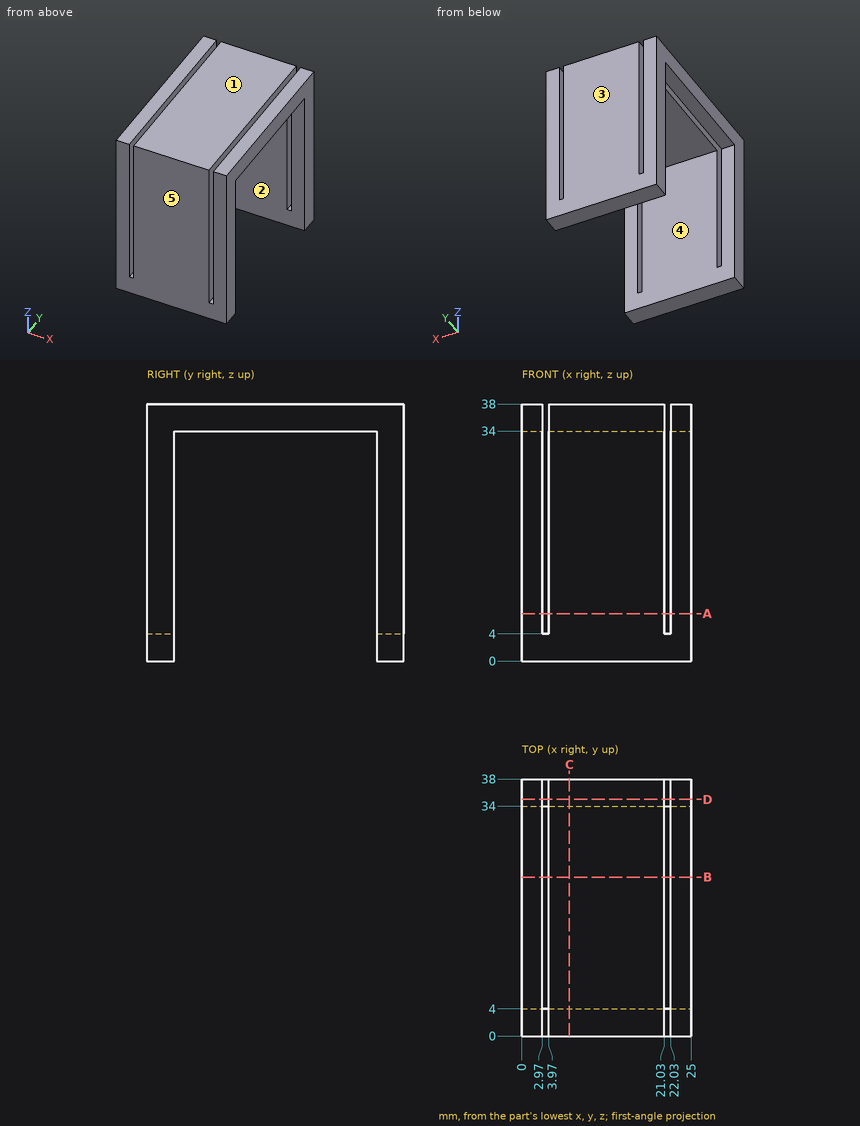
Part print with two shaded views. Sizes in mm from the minimum x, y, z corner. A direction names the side the tool comes from. Coordinates: 2 decimals unless noted, no trailing zeros. Write each loop counter-clockwise with the first axis right and the second up, starting at its lowest first coordinate (ties: lowest second). Pieces come first, ordered by that corner, then holes. Notation, with made-up numbers: (34, 62) - (41, 62) arc R24 cw to (41, 81) - close; hole circle Ø3 at (75, 76). An arc over 180 degrees is marked (long way). One line per item, written item: value. Start each with the question number.
1. Flat gauge pins, fed straight in: pin 1 (3.5 mm diameter, centred on x = 2, y = 20.5, fed in from -Z); pin 2 (0.8 mm diameter, centred on x = 21.5, y = 35, fed in from +Z); pin 3 (10 mm diameter, centred on y = 28, z = 23.5, fed in from -X). Where does each tip first touch, or does it go through?
2. Slice it at D-D (y = 35). Write the cut outline in (x, z).
3. Mould opens along Y. For the marked faces 3, 4 and 5 say: released by +Y, released by -Y, zero draft, split by the parting line, or undercut.
4. Slice it at C-C (x = 7). Write the cut outline in (y, z), plus the area to 3 significant figures.
5. Slice it at A-A (z = 7). Write the cut outline in (x, y), plus the area to 3 significant figures.
6. Probe line 1 (X direction, y = 35.5, z = 5); line 2 (Y direction, x = 14.25, z = 3.5); line 3 (Z direction, x = 15.25, y = 18). List the from-to ranges inside material, lowest first. Write a range as from..to.
7. Tool access for the marked faces 1 and 2: list every direction of +Z, -Z, +X, -X, +Y, -Y with a clear straight run to the whole face (end or side of a thin tool).
8. Slice it at B-B (y = 23.5). Write the cut outline in (x, z), plus the area to 3 significant figures.
Answers below:
1. pin 1: stops at z = 34
1. pin 2: stops at z = 4
1. pin 3: passes through
2. outline: (0, 0) - (25, 0) - (25, 38) - (22.03, 38) - (22.03, 4) - (21.03, 4) - (21.03, 38) - (3.97, 38) - (3.97, 4) - (2.97, 4) - (2.97, 38) - (0, 38) - close
3. face 3: released by +Y
3. face 4: undercut
3. face 5: released by -Y
4. outline: (0, 0) - (4, 0) - (4, 34) - (34, 34) - (34, 0) - (38, 0) - (38, 38) - (0, 38) - close
4. area: 424 mm^2
5. outline: (0, 0) - (2.97, 0) - (2.97, 4) - (0, 4) - close; (0, 34) - (2.97, 34) - (2.97, 38) - (0, 38) - close; (3.97, 0) - (21.03, 0) - (21.03, 4) - (3.97, 4) - close; (3.97, 34) - (21.03, 34) - (21.03, 38) - (3.97, 38) - close; (22.03, 0) - (25, 0) - (25, 4) - (22.03, 4) - close; (22.03, 34) - (25, 34) - (25, 38) - (22.03, 38) - close
5. area: 184 mm^2
6. line 1: x = 0..2.97, 3.97..21.03, 22.03..25
6. line 2: y = 0..4, 34..38
6. line 3: z = 34..38
7. face 1: +Z, +X, -X, +Y, -Y
7. face 2: -Z, +X, -X
8. outline: (0, 34) - (2.97, 34) - (2.97, 38) - (0, 38) - close; (3.97, 34) - (21.03, 34) - (21.03, 38) - (3.97, 38) - close; (22.03, 34) - (25, 34) - (25, 38) - (22.03, 38) - close
8. area: 92.0 mm^2
